Part model, mm, in its own coordinate system. A direction names the side the tool comes from. Round coordinates to 2 decimals unless told otherwise and drop trailing zeros. Loops run counter-clockwise (first coordinate to the right, second up) from the corner with the lowest first, then second, coordinate; pieces in that order, holes last.
(1) Cut at B-B on y = -5. Count the separate pieces of the cut face and the enclosed holes in it, then the cut area to 3 significant figures.
(2) Cut at D-D on z = -2. List the corners of the cut face in (x, y), then the cut area to 3 significant figures.
(3) Cut at A-A on x = 21.5. List the corners of the cut face in (y, z), then the cut area to 3 significant figures.
(4) Flat gauge pins, fed straight in: pin 1 (1.6 mm diameter, centred on y = -14, z = 1.5, fed in from -X); pin 2 (5 mm diameter, centred on x = -4, y = -3.5, fed in from -Z); pin 3 (2 mm diameter, centred on x = 18, z = -1.5, fed in from -Y). Where does each tip first touch, or does it go through?
(5) Mould opens along X. For faces 1 (the face through (-3, -5, 1)), 2 (the face through (9.77, -3.85, 0.99)), 3 (the face through (36.5, -4, -1)), 4 (the face through (80, -10.5, 1)) say: +X half, -X half, draft (parallel to the pull), parting line (faces both ways), or undercut.
(6) Probe probe 1 along X at (y, z) = (-19.5, 1.5); probe 2 along X at (y, z) = (-5, 1.55); probe 3 along X at (y, z) = (-13.75, 1.45). List the from-to ranges inside material, lowest first.
(7) Tool access for faces 5 (the face through (70, -8.5, -1)), 6 (the face through (25.7, -19.1, 1)), 7 (the face through (38.5, -3, -1)): list every direction of +Z, -Z, +X, -X, +Y, -Y with a clear straight run to the whole face (end or side of a thin tool).
(8) Cut at C-C on y = -19.5. List the corners of the cut face in (x, z), then the cut area to 3 significant figures.
from build123d import *

# Parameters (mm, degrees)
SKETCH_R        = 2.5
PAD_DEPTH       = 2
PAD001_DEPTH    = 3
SKETCH004_W     = 6
SKETCH004_H     = 10
SKETCH004_W_2   = 8
SKETCH004_H_2   = 11
SKETCH004_W_3   = 10
POCKET_DEPTH    = 1
SKETCH005_R     = 3
SKETCH005_R_2   = 1.5
POCKET001_DEPTH = 5


with BuildPart() as part:
    # Sketch → Pad (new body)
    with BuildSketch(Plane.XY):
        Polygon((0, 0), (-6, 0), (-6, -10), (0, -10), (4, -13.5), (23.566, -13.5), (23.566, -24.5), (31.566, -24.5), (31.566, -13.5), (62, -13.5), (62, -24.5), (72, -24.5), (72, -13.5), (75, -13.5), (75, -18.5), (78, -18.5), (78, -10.5), (83, -10.5), (83, -18.5), (86, -18.5), (86, 0.5), (71, 0.5), (71, 3.5), (4, 3.5), align=None)
        with Locations((28.566, -19.5)):
            Circle(SKETCH_R, mode=Mode.SUBTRACT)
        with Locations((67, -19.5)):
            Circle(SKETCH_R, mode=Mode.SUBTRACT)
    extrude(amount=PAD_DEPTH)

    # Sketch003 (on Face27 of Pad) → Pad001 (join)
    with BuildSketch(Plane(origin=(0, 0, 0), x_dir=(1, 0, 0), z_dir=(0, 0, -1))):
        Polygon((6, -3.5), (71, -3.5), (71, 8.5), (69, 8.5), (69, -1.5), (38.5, -1.5), (38.5, 8.5), (36.5, 8.5), (36.5, -1.5), (6, -1.5), align=None)
    extrude(amount=PAD001_DEPTH)

    # Sketch004 (on Face4 of Pad001) → Pocket (cut)
    with BuildSketch(Plane(origin=(0, 0, 0), x_dir=(1, 0, 0), z_dir=(0, 0, -1))):
        with Locations((-3, 5)):
            Rectangle(SKETCH004_W, SKETCH004_H)
        with Locations((27.566, 19)):
            Rectangle(SKETCH004_W_2, SKETCH004_H_2)
        with Locations((67, 19)):
            Rectangle(SKETCH004_W_3, SKETCH004_H_2)
    extrude(amount=-POCKET_DEPTH, mode=Mode.SUBTRACT)

    # Sketch005 (on Face4 of Pocket) → Pocket001 (cut)
    with BuildSketch(Plane(origin=(0, 0, 0), x_dir=(1, 0, 0), z_dir=(0, 0, -1))):
        with Locations((7, 5)):
            Circle(SKETCH005_R)
        with Locations((13.5, 5)):
            Circle(SKETCH005_R_2)
        with Locations((21.5, 5)):
            Circle(SKETCH005_R)
        with Locations((28, 5)):
            Circle(SKETCH005_R_2)
    extrude(amount=-POCKET001_DEPTH, mode=Mode.SUBTRACT)


solid = part.part
Final values:
1. separate pieces: 5
1. enclosed holes: 0
1. area: 154 mm2
2. outline: (6, 1.5) - (36.5, 1.5) - (36.5, -8.5) - (38.5, -8.5) - (38.5, 1.5) - (69, 1.5) - (69, -8.5) - (71, -8.5) - (71, 3.5) - (6, 3.5) - close
2. area: 170 mm2
3. outline: (-13.5, 0) - (-8, 0) - (-8, 2) - (-13.5, 2) - close; (-2, 0) - (1.5, 0) - (1.5, -3) - (3.5, -3) - (3.5, 2) - (-2, 2) - close
3. area: 28.0 mm2
4. pin 1: stops at x = 3.66
4. pin 2: stops at z = 1
4. pin 3: stops at y = 1.5
5. face 1: draft
5. face 2: undercut
5. face 3: -X half
5. face 4: undercut
6. probe 1: x = 23.57 to 26.07, 31.07 to 31.57, 62 to 64.5, 69.5 to 72
6. probe 2: x = -6 to 4, 10 to 12, 15 to 18.5, 24.5 to 26.5, 29.5 to 86
6. probe 3: x = 23.57 to 31.57, 62 to 72, 75 to 78, 83 to 86
7. face 5: -Z, +X, -X, -Y
7. face 6: -Z, -X, -Y
7. face 7: -Z, -Y
8. outline: (23.57, 1) - (26.07, 1) - (26.07, 2) - (23.57, 2) - close; (31.07, 1) - (31.57, 1) - (31.57, 2) - (31.07, 2) - close; (62, 1) - (64.5, 1) - (64.5, 2) - (62, 2) - close; (69.5, 1) - (72, 1) - (72, 2) - (69.5, 2) - close
8. area: 8.00 mm2
